Check sheet for the modelled part. Datum: model origin and axes. Units: mm. Face numbers are marked on the shaded views. Coordinates: 2 decimals unless noted, no trailing zeros. Loops run counter-clockwise (first coordinate to the right, second up) from the corner with the lowest first, then second, coordinate; pieces in that order, holes last. Notation, with made-up numbers: M 63.25,51 L 93.25,51 A17 ccw 93.25,66 Z; hole C 75,24 d10. An arc over 180 degrees is marked long. Answer as CSV lines item,"result". Start each with the question number.
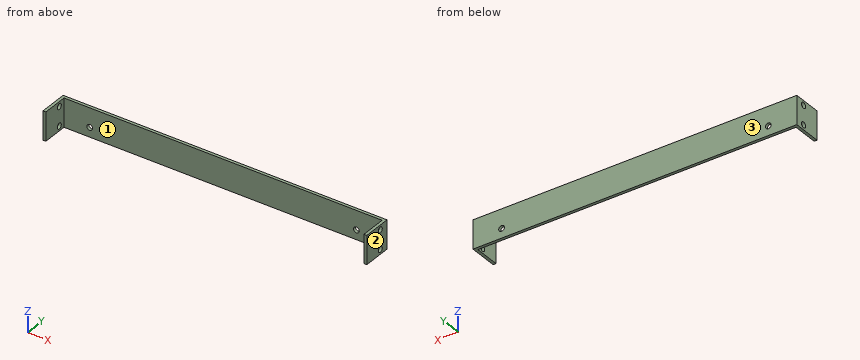
from build123d import *

# Parameters (mm, degrees)
SKETCH1_W               = 167
SKETCH1_H               = 15
BOSS_EXTRUDE1_DEPTH     = 1.5
SKETCH2_W               = 15
SKETCH2_H               = 15
BOSS_EXTRUDE2_DEPTH     = 1.5
SKETCH3_W               = 15
SKETCH3_H               = 15
BOSS_EXTRUDE3_DEPTH     = 1.5
SKETCH5_R               = 1.5
CUT_EXTRUDE1_DEPTH      = 1000
CUT_EXTRUDE1_DEPTH_BACK = 10000
SKETCH4_R               = 1.5
CUT_EXTRUDE2_DEPTH      = 10000
CUT_EXTRUDE2_DEPTH_BACK = 10000


with BuildPart() as part:
    # Sketch1 → Boss-Extrude1 (new body)
    with BuildSketch(Plane(origin=(0, 0, 0), x_dir=(1, 0, 0), z_dir=(0, 1, 0))):
        with Locations((83.5, 7.5)):
            Rectangle(SKETCH1_W, SKETCH1_H)
    extrude(amount=BOSS_EXTRUDE1_DEPTH)

    # Sketch2 → Boss-Extrude2 (add)
    with BuildSketch(Plane(origin=(167, 0, 0), x_dir=(0, 0, -1), z_dir=(1, 0, 0))):
        with Locations((7.5, -6)):
            Rectangle(SKETCH2_W, SKETCH2_H)
    extrude(amount=BOSS_EXTRUDE2_DEPTH)

    # Sketch3 → Boss-Extrude3 (add)
    with BuildSketch(Plane.ZY):
        with Locations((-7.5, -6)):
            Rectangle(SKETCH3_W, SKETCH3_H)
    extrude(amount=BOSS_EXTRUDE3_DEPTH)

    # Sketch5 → Cut-Extrude1 (cut, two sides)
    with BuildSketch(Plane(origin=(168.5, 0, 0), x_dir=(0, 0, -1), z_dir=(1, 0, 0))) as cut_extrude1_sk:
        with Locations((2.5, -3.5)):
            Circle(SKETCH5_R)
        with Locations((12.5, -3.5)):
            Circle(SKETCH5_R)
    extrude(amount=CUT_EXTRUDE1_DEPTH, mode=Mode.SUBTRACT)
    extrude(cut_extrude1_sk.sketch, amount=-CUT_EXTRUDE1_DEPTH_BACK, mode=Mode.SUBTRACT)

    # Sketch4 → Cut-Extrude2 (cut, two sides)
    with BuildSketch(Plane(origin=(0, 1.5, 0), x_dir=(1, 0, 0), z_dir=(0, 1, 0))) as cut_extrude2_sk:
        with Locations((13.5, 10)):
            Circle(SKETCH4_R)
        with Locations((153.5, 10)):
            Circle(SKETCH4_R)
    extrude(amount=CUT_EXTRUDE2_DEPTH, mode=Mode.SUBTRACT)
    extrude(cut_extrude2_sk.sketch, amount=-CUT_EXTRUDE2_DEPTH_BACK, mode=Mode.SUBTRACT)


solid = part.part
Item 1: Sectioned sample at B-B, the plane x = 13.5. Record the boundary of the cut face in (y, z).
Item 2: Sectioned sample at A-A, the plane y = -6.5. Record the boundary of the cut face in (x, z), and give its area (3 significant figures).
Item 3: Material ranges on line 1 (X direction, y = 0.45, z = -10); line 2 (X direction, y = -5, z = -13.5); line 3 (Y direction, x = -0.4, z = -12.5), recorded low to high. Write a range as from..to.
Item 4: Go/stop test with flat-tipped pins: pin 1 (1.8 mm diameter, centred on y = -3.5, z = -12.5, fed in from -X); pin 2 (3.5 mm diameter, centred on x = 153.5, z = -10, fed in from -Y). Record where each tip stops, or that it passes through.
Item 5: Release check for a two-part mould opening along X. For the marked faces 1, 2 and 3 record: released by +X, released by -X, zero draft, split by the parting line, or undercut.
Reply:
1,outline,"M 0,-15 L 1.5,-15 L 1.5,-11.5 L 0,-11.5 Z; M 0,-8.5 L 1.5,-8.5 L 1.5,0 L 0,0 Z"
2,outline,"M -1.5,-15 L 0,-15 L 0,0 L -1.5,0 Z; M 167,-15 L 168.5,-15 L 168.5,0 L 167,0 Z"
2,area,"45.0 mm²"
3,line 1,"-1.5..12, 15..152, 155..168.5"
3,line 2,"-1.5..0, 167..168.5"
3,line 3,"-13.5..-5, -2..1.5"
4,pin 1,"through"
4,pin 2,"y = 0"
5,face 1,"undercut"
5,face 2,"released by +X"
5,face 3,"zero draft"
